Build history of the part. All positions in model axes, mm. A direction names the side the tool comes from. Round coordinates to 2 decimals unless told otherwise and drop trailing zeros. Loops run counter-clockwise (first coordinate to the right, second up) from the corner with the lowest first, then second, coordinate; pieces in that order, holes last. Notation, with made-up numbers: (48.25, 7) - (90.25, 7) arc R34 ccw to (90.25, 41) - close; hole circle Ø11 at (40.5, -15). An arc over 180 degrees is marked (long way). Use one line per item in the form item = value. Start each with the question number.
Q1. 3-axis set-ups, long thin cutter, end or side, ignore diameter. For faces 5 (the face through (-3, -7, 2)), 6 (the face through (3.1, 1.2, 1.6)), 7 (the face through (-2.5, 9, 2)): which of +Z, -Z, +X, -X, +Y, -Y reach the whole face in a straight line?
Q2. Mould opens along X. For faces 1 (the face through (3, -7, 2)), 2 (the face through (-3.1, 1.2, 1.6)), 3 (the face through (-1.75, -10, 2)), 4 (the face through (6, -5, 2)) say: released by +X, released by -X, zero draft, split by the parting line, or undercut.
Q3. Saw through at B-B (x = -1.25). Give the cut face in (y, z).
Q4. Saw through at D-D (y = 2.25). Give the cut face in (x, z), then the cut area to 3 significant figures.
Q5. Pin check, flat tips, straight feed: pin 1 (0.5 mm diameter, centred on x = 2.5, z = 2, fed in from +Y); pin 2 (0.8 mm diameter, centred on x = 1, z = 2.5, fed in from -Y); pin 3 (0.5 mm diameter, centred on y = -9.5, z = 1.5, fed in from -X); pin 4 (3 mm diameter, centred on x = -4.5, y = 5, fed in from +Z). Stop position of each tip, or through.
Q6. Drill centre lines: line 1 (X direction, y = -6, z = 2.4); line 2 (Y direction, x = -0.75, z = 0.95); line 3 (X direction, y = 3.75, z = 1.3). Where is each one in solid material? Low to high.
Q7. Saw through at C-C (y = 11.75). Give the cut face in (x, z), then the cut area to 3 significant figures.
Q8. Saw through at A-A (y = -7.5). Give the cut face in (x, z).
Autodesk Fusion 360 part; units mm, degrees
sketch "スケッチ1" plane through (0, 0, 0) normal (0, 0, 1) x (1, 0, 0)
  line L0 (-6, -10.8) -> (-1.75, -10.8)
  line L1 (-1.75, -10.8) -> (-1.75, -9.3)
  line L2 (-1.75, -9.3) -> (-3, -9.3)
  line L3 (-3, -9.3) -> (-3, -5)
  line L4 (-3, -5) -> (3, -5)
  line L5 (3, -5) -> (3, -9.3)
  line L6 (3, -9.3) -> (1.75, -9.3)
  line L7 (1.75, -9.3) -> (1.75, -10.8)
  line L8 (1.75, -10.8) -> (6, -10.8)
  line L9 (6, -10.8) -> (6, 0)
  line L10 (6, 0) -> (5.5, 0)
  line L11 (2.5, 3) -> (2.5, 15)
  line L12 (2.5, 15) -> (-2.5, 15)
  line L13 (-2.5, 15) -> (-2.5, 3)
  line L14 (-5.5, 0) -> (-6, 0)
  line L15 (-6, 0) -> (-6, -10.8)
  line L16 (0, 0) -> (0, -5) construction
  line L17 (-2.5, 0) -> (1.5, 0) construction
  arc A0 (-5.5, 0) -> (-2.5, 3) centre (-5.5, 3) ccw
  arc A1 (2.5, 3) -> (5.5, 0) centre (5.5, 3) ccw
  dimension "d4" = 6
  dimension "d5" = 1.5
  dimension "d6" = 4.3
  dimension "d7" = 3
  dimension "d8" = 5
  dimension "d9" = 5
  dimension "d10" = 15
  dimension "d11" = 3.5
  dimension "d12" = 3
  dimension "d13" = 3
extrude "押し出し1" add sketch "スケッチ1" along normal blind 3.2
fillet "フィレット1" radius 2 4 edges at (-6, 0, 1.6) (-6, -10.8, 1.6) (6, 0, 1.6) (6, -10.8, 1.6)
chamfer "面取り1" distance 1 angle 45 2 edges at (2.5, 15, 1.6) (-2.5, 15, 1.6)
chamfer "面取り2" distance 0.5 angle 45 2 edges at (1.75, -10.8, 1.6) (-1.75, -10.8, 1.6)
chamfer "面取り3" distance 0.4 angle 45 3 edges at (3, -7.15, 0) (0, -5, 0) (-3, -7.15, 0)
equation "d1 = 3.7 mm - 0.5 mm"
Report:
q1.face_5 = +Z, -Z
q1.face_6 = +Z, -Z, +X, +Y
q1.face_7 = +Z, -Z, -X, +Y
q2.face_1 = undercut
q2.face_2 = released by -X
q2.face_3 = undercut
q2.face_4 = released by +X
q3.outline = (-5, 0.4) - (-4.6, 0) - (15, 0) - (15, 3.2) - (-5, 3.2) - close
q4.outline = (-2.6, 0) - (2.6, 0) - (2.6, 3.2) - (-2.6, 3.2) - close
q4.area = 16.6 mm²
q5.pin_1 = 14.25
q5.pin_2 = -5
q5.pin_3 = -5.95
q5.pin_4 = through
q6.line_1 = -6 to -3, 3 to 6
q6.line_2 = -5 to 15
q6.line_3 = -2.5 to 2.5
q7.outline = (-2.5, 0) - (2.5, 0) - (2.5, 3.2) - (-2.5, 3.2) - close
q7.area = 16.0 mm²
q8.outline = (-6, 0) - (-3.4, 0) - (-3, 0.4) - (-3, 3.2) - (-6, 3.2) - close; (3, 0.4) - (3.4, 0) - (6, 0) - (6, 3.2) - (3, 3.2) - close
